Input: part model. Units: mm. Frame: model coordinates. A direction names the side the tool comes from. Give positions to 0.01 mm unless a question says otherwise; leave off trailing zeros. Loops run counter-clockwise (first coordinate to the right, second up) from the corner with the lowest first, then second, coordinate; pieces in that order, holes last.
from build123d import *

# Parameters (mm, degrees)
SKETCH1_W                       = 101.6
SKETCH1_H                       = 88.9
BOSS_EXTRUDE1_DEPTH             = 9.525
F_8_32_TAPPED_HOLE1_D           = 3.4544
F_8_32_TAPPED_HOLE1_DEPTH       = 19.05
F_8_32_TAPPED_HOLE1_CSINK_D     = 4.1656
F_8_32_TAPPED_HOLE1_CSINK_ANGLE = 90
F_8_32_TAPPED_HOLE1_TIP         = 1.037806461
F_8_CLEARANCE_HOLE2_D           = 4.4958
F_8_CLEARANCE_HOLE2_DEPTH       = 25.4
F_8_CLEARANCE_HOLE2_TIP         = 1.350674586
F_6_32_TAPPED_HOLE1_D           = 2.7051
F_4_CLEARANCE_HOLE1_D           = 3.2639
F_4_CLEARANCE_HOLE1_DEPTH       = 9.525
F_4_CLEARANCE_HOLE2_D           = 3.2639
F_4_CLEARANCE_HOLE2_DEPTH       = 9.525


with BuildPart() as part:
    # Sketch1 → Boss-Extrude1 (new body)
    with BuildSketch(Plane.XY):
        with Locations((-50.8, 44.45)):
            Rectangle(SKETCH1_W, SKETCH1_H)
    extrude(amount=BOSS_EXTRUDE1_DEPTH)

    # #8-32 Tapped Hole1
    with Locations(Plane(origin=(0, 88.9, 0), x_dir=(1, 0, 0), z_dir=(0, 1, 0))):
        with Locations((-44.45, -4.7625), (-57.15, -4.7625)):
            CounterSinkHole(F_8_32_TAPPED_HOLE1_D / 2, F_8_32_TAPPED_HOLE1_CSINK_D / 2, depth=F_8_32_TAPPED_HOLE1_DEPTH, counter_sink_angle=F_8_32_TAPPED_HOLE1_CSINK_ANGLE)
            with Locations((0, 0, -(F_8_32_TAPPED_HOLE1_DEPTH + F_8_32_TAPPED_HOLE1_TIP / 2))):  # 118° drill point
                Cone(0, F_8_32_TAPPED_HOLE1_D / 2, F_8_32_TAPPED_HOLE1_TIP, mode=Mode.SUBTRACT)

    # #8 Clearance Hole2
    with Locations(Plane.XY.offset(9.525)):
        with Locations((-44.45, 68.812193539), (-57.15, 68.812193539)):
            Hole(F_8_CLEARANCE_HOLE2_D / 2, depth=F_8_CLEARANCE_HOLE2_DEPTH)
            with Locations((0, 0, -(F_8_CLEARANCE_HOLE2_DEPTH + F_8_CLEARANCE_HOLE2_TIP / 2))):  # 118° drill point
                Cone(0, F_8_CLEARANCE_HOLE2_D / 2, F_8_CLEARANCE_HOLE2_TIP, mode=Mode.SUBTRACT)

    # #6-32 Tapped Hole1 (through all)
    with Locations(Plane.XY.offset(9.525)):
        with Locations((-95.25, 6.35), (-95.25, 82.55), (-6.35, 6.35), (-6.35, 82.55)):
            Hole(F_6_32_TAPPED_HOLE1_D / 2)

    # #4 Clearance Hole1
    with Locations(Plane.XY.offset(9.525)):
        with Locations((-17.4625, 10.033), (-84.1375, 10.033)):
            Hole(F_4_CLEARANCE_HOLE1_D / 2, depth=F_4_CLEARANCE_HOLE1_DEPTH)

    # #4 Clearance Hole2
    with Locations(Plane(origin=(0, 0, 0), x_dir=(-1, 0, 0), z_dir=(0, 0, -1))):
        with Locations((23.368, 41.275), (78.232, 41.275)):
            Hole(F_4_CLEARANCE_HOLE2_D / 2, depth=F_4_CLEARANCE_HOLE2_DEPTH)


solid = part.part
(1) Cut plane A-A (x = -95.25). Return the cut outline in (y, z) (3 decimals), and give its area (3 significant figures).
Values follow:
outline: (0, 0) - (4.997, 0) - (4.997, 9.525) - (0, 9.525) - close; (7.703, 0) - (81.197, 0) - (81.197, 9.525) - (7.703, 9.525) - close; (83.903, 0) - (88.9, 0) - (88.9, 9.525) - (83.903, 9.525) - close
area: 795 mm2
(2) Reachability of faces 1 (the cylindrical face through (-43.177, 79.27, 3.595)), 2 (the cylindrical face through (-94.96, 81.23, 4.7)) from +Z, -Z, +X, -X, +Y, -Y: full face, straight path, thin tool, end or side. Return the list, or none.
Values follow:
face 1: +Y
face 2: +Z, -Z
(3) Cut plane C-C (x = -84.5). Return the cut outline in (y, z) (3 decimals).
Values follow:
outline: (0, 0) - (8.442, 0) - (8.442, 9.525) - (0, 9.525) - close; (11.624, 0) - (88.9, 0) - (88.9, 9.525) - (11.624, 9.525) - close
(4) Ray query, probe 1 along X at (y, z) = (75.5, 4.75); probe 2 along Z at (x, y) = (-57.15, 80) (3 decimals); probe 3 along X at (y, z) = (82.55, 5.5). Return the intervals inside material, ascending.
Values follow:
probe 1: x = -101.6 to -58.88, -55.42 to -46.18, -42.72 to 0
probe 2: z = 0 to 3.035, 6.49 to 9.525
probe 3: x = -101.6 to -96.6, -93.9 to -58.71, -55.59 to -46.01, -42.89 to -7.7, -5 to 0
(5) Cut plane D-D (x = -44.45). Return the cut outline in (y, z) (3 decimals).
Values follow:
outline: (0, 0) - (66.564, 0) - (66.564, 9.525) - (0, 9.525) - close; (71.06, 0) - (88.9, 0) - (88.9, 2.68) - (88.544, 3.035) - (71.06, 3.035) - close; (71.06, 6.49) - (88.544, 6.49) - (88.9, 6.845) - (88.9, 9.525) - (71.06, 9.525) - close
(6) Cut plane B-B (y = 6.35). Return the cut outline in (x, z) (3 decimals), and give its area (3 significant figures).
Values follow:
outline: (-101.6, 0) - (-96.603, 0) - (-96.603, 9.525) - (-101.6, 9.525) - close; (-93.897, 0) - (-7.703, 0) - (-7.703, 9.525) - (-93.897, 9.525) - close; (-4.997, 0) - (0, 0) - (0, 9.525) - (-4.997, 9.525) - close
area: 916 mm2
(7) Pin query (flat end, axial travel): pin 1 Ø2 at (x, z) = (-57.15, 4.76) entering from +Y. Return the tip coordinate at first contact, or that it passes through.
Values follow:
pin 1: stops at y = 66.8
(8) Mould query, pull axis Y, two halves, no side actions, for faces 3 (the flat face through (-52, 0, 5)), 4 (the cylindrical face through (-82.507, 10.105, 4.696)), 5 (the flat face through (-52, 45, 0)). Classes: +Y half, -Y half, draft (parallel to the pull), parting line (faces both ways), or undercut.
Values follow:
face 3: -Y half
face 4: undercut
face 5: draft
